Design review of the part built by this model. Coordinates are the model's own, in mm. Face numbers are marked on the shaded views. Coordinates: 2 decimals unless noted, no trailing zeros. Loops run counter-clockwise (first coordinate to the right, second up) from the corner with the lowest first, then second, coordinate; pieces in that order, holes last. Notation, with made-up numbers: (-19.5, 29.5) - (-13.5, 29.5) arc R24 cw to (-13.5, 58.5) - close; hole circle Ø4 at (67.25, 24). An arc over 180 degrees is marked (long way). Use one line per item in the form item = value. Start each with the question number.
(1) Clearance check with flat-ended pins moving along their axes: pin 1 Ø10 at (x, y) = (608.5, 25) entering from -Z; pin 2 Ø1 at (x, z) = (461, -40.5) entering from -Y; pin 3 Ø4 at (x, y) = (582.5, 4.5) entering from +Z. State where each tip first meets the part, or that it passes through.
(2) The part is to be moulded in two halves that separate along Z. For the marked faces 1 and 2, say which applies: pulls with the +Z half, pulls with the -Z half, needs draft (parallel to the pull), parting line crosses it, or undercut.
(3) For L1, parallel to Y at x = 491, z = 0; L2, parallel to Y at x = 541, z = -16; L3, parallel to Z at x = 656, y = 26, list the stretches that pass through material, from the lowest coordinate up.
(4) Add section A-A (z = 0). State the section outline as (x, y) points, plus the area to 3 significant figures.
(5) Add section C-C (x = 515). State the section outline as (y, z) points, plus the area to 3 significant figures.
```python
from build123d import *

# Parameters (mm, degrees)
SKETCH1_R           = 60.75
SKETCH1_R_2         = 52.75
BOSS_EXTRUDE1_DEPTH = 750
FILLET1_R           = 2
FILLET2_R           = 2


with BuildPart() as part:
    # Sketch1 → Boss-Extrude1 (new body)
    with BuildSketch(Plane(origin=(0, 0, 0), x_dir=(0, 0, -1), z_dir=(1, 0, 0))):
        Circle(SKETCH1_R)
        Circle(SKETCH1_R_2, mode=Mode.SUBTRACT)
    extrude(amount=BOSS_EXTRUDE1_DEPTH)

    # Fillet1
    fillet1_edges = [part.edges().sort_by_distance(p)[0] for p in [
        (750, 0, 60.75),
        (750, 0, 52.75),
    ]]
    fillet(fillet1_edges, radius=FILLET1_R)

    # Fillet2
    fillet2_edges = [part.edges().sort_by_distance(p)[0] for p in [
        (0, 0, 60.75),
        (0, 0, 52.75),
    ]]
    fillet(fillet2_edges, radius=FILLET2_R)


solid = part.part
```
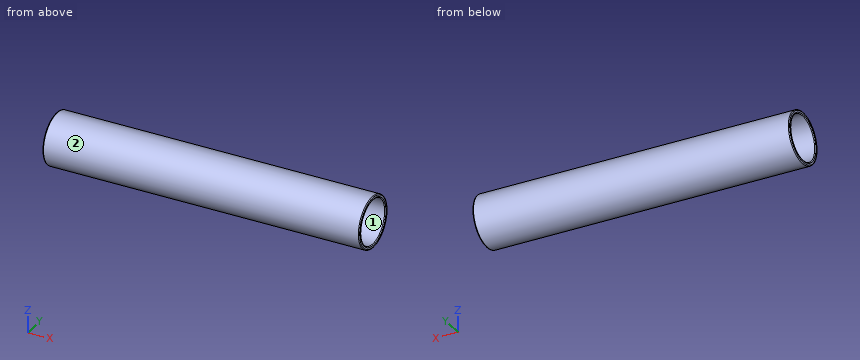
Computed values:
q1.pin_1 = -57.36
q1.pin_2 = -45.72
q1.pin_3 = 60.7
q2.face_1 = undercut
q2.face_2 = parting line crosses it
q3.L1 = -60.75 to -52.75, 52.75 to 60.75
q3.L2 = -58.61 to -50.26, 50.26 to 58.61
q3.L3 = -54.91 to -45.9, 45.9 to 54.91
q4.outline = (0, -58.75) arc R2 ccw to (2, -60.75) - (748, -60.75) arc R2 ccw to (750, -58.75) - (750, -54.75) arc R2 ccw to (748, -52.75) - (2, -52.75) arc R2 ccw to (0, -54.75) - close; (0, 54.75) arc R2 ccw to (2, 52.75) - (748, 52.75) arc R2 ccw to (750, 54.75) - (750, 58.75) arc R2 ccw to (748, 60.75) - (2, 60.75) arc R2 ccw to (0, 58.75) - close
q4.area = 12,000 mm^2
q5.outline = circle Ø121.5 at (0, 0); hole circle Ø105.5 at (0, 0)
q5.area = 2,850 mm^2
